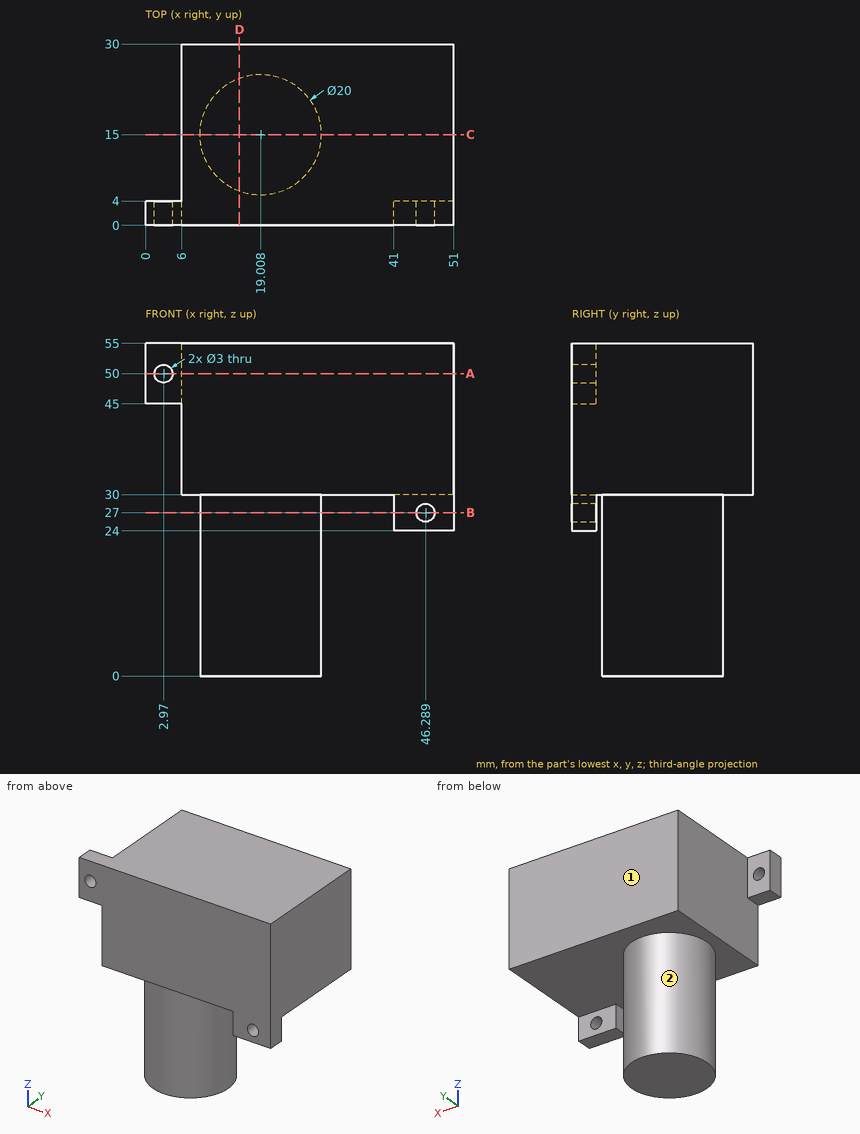
Input: dimensioned drawing with shaded views. Units: mm. Origin: part minimum x, y, z. A direction names the side the tool comes from. Coordinates: 2 decimals unless noted, no trailing zeros. Loops run counter-clockwise (first coordinate to the right, second up) from the corner with the lowest first, then second, coordinate; pieces in that order, holes last.
Q1. Section A-A, the plane z = 50. Return the cut outline in (x, y), and give its area (3 significant figures).
Results are:
outline: (0, 0) - (1.47, 0) - (1.47, 4) - (0, 4) - close; (4.47, 0) - (51, 0) - (51, 30) - (6, 30) - (6, 4) - (4.47, 4) - close
area: 1,360 mm2
Q2. Section D-D, the plane x = 15.5. Return the cut outline in (y, z) (1 decimal).
Results are:
outline: (0, 30) - (5.6, 30) - (5.6, 0) - (24.4, 0) - (24.4, 30) - (30, 30) - (30, 55) - (0, 55) - close
Q3. Contact query for flat-ended pins moving along their axis: pin 1 (10 mm diameter, centred on y = 18.5, z = 43, fed in from -X); pin 2 (6.5 mm diameter, centred on x = 1.5, z = 48.5, fed in from +Y); pin 3 (2 mm diameter, centred on y = 1.5, z = 26.5, fed in from -X); pin 4 (2.5 mm diameter, centred on x = 46.29, z = 27, fed in from +Y). Output: stop coordinate, or through.
Results are:
pin 1: stops at x = 6
pin 2: stops at y = 4
pin 3: stops at x = 41
pin 4: passes through
Q4. Section B-B, the plane z = 27. Return the cut outline in (x, y), and give its area (3 significant figures).
Results are:
outline: circle Ø20 at (19.01, 15); (41, 0) - (44.79, 0) - (44.79, 4) - (41, 4) - close; (47.79, 0) - (51, 0) - (51, 4) - (47.79, 4) - close
area: 342 mm2
Q5. Set-up query: the marked faces 1 and 2. Return all of +Z, -Z, +X, -X, +Y, -Y with unobstructed straight access to the full face (end or side cutting, diameter ignored); none if empty.
Results are:
face 1: +Z, -Z, +X, -X, +Y
face 2: -Z
Q6. Line query: line 1 along X through (y, z) = (1.35, 27); line 2 along X through (y, z) = (1.15, 50); line 3 along Z through (x, y) = (30, 22.75). Output: solid intervals per line, ascending.
Results are:
line 1: x = 41 to 44.79, 47.79 to 51
line 2: x = 0 to 1.47, 4.47 to 51
line 3: z = 30 to 55
Q7. Section C-C, the plane y = 15. Return the cut outline in (x, z), and give its area (4 significant figures).
Results are:
outline: (6, 30) - (9.01, 30) - (9.01, 0) - (29.01, 0) - (29.01, 30) - (51, 30) - (51, 55) - (6, 55) - close
area: 1,725 mm2
